Read the model definition and answer for the solid it produces. Units are mm, in the model's axes. Face numbers are marked on the shaded views. A direction names the side the tool comes from. Coordinates: 2 decimals unless noted, no trailing zeros. Order: outer loops, then holes, each group sorted by start corner. A loop starts at its lowest first (then second) coordinate and runs counter-clockwise, first axis right, second up. Notation, with made-up numbers: (21.25, 6.5) - (38.25, 6.5) arc R33 cw to (38.25, 42.5) - close; hole circle Ø4 at (79, -28.75). An arc over 180 degrees is marked (long way). Use one line per item in the form item = value.
```python
from build123d import *

# Parameters (mm, degrees)
BOSS_EXTRUDE2_DEPTH = 20
SKETCH2_R           = 3
CUT_EXTRUDE1_DEPTH  = 20
SKETCH3_W           = 200
SKETCH3_H           = 120
CUT_EXTRUDE2_DEPTH  = 10
FILLET1_R           = 5
BOSS_EXTRUDE3_START = -10
SKETCH6_R           = 3
SKETCH6_R_2         = 2.5
BOSS_EXTRUDE3_DEPTH = 10
SKETCH7_R           = 4.7
CUT_EXTRUDE6_DEPTH  = 5
SKETCH4_W           = 18
SKETCH4_H           = 81
CUT_EXTRUDE7_DEPTH  = 5


with BuildPart() as part:
    # Sketch1 → Boss-Extrude2 (new body)
    with BuildSketch(Plane.XY):
        Polygon((0, 0), (240, 0), (240, 10), (220, 10), (220, 130), (20, 130), (20, 10), (0, 10), align=None)
    extrude(amount=BOSS_EXTRUDE2_DEPTH)

    # Sketch2 → Cut-Extrude1 (cut)
    with BuildSketch(Plane(origin=(0, 10, 0), x_dir=(1, 0, 0), z_dir=(0, 1, 0))):
        with Locations(Location((10, -10, 0), (0, 0, 180))):
            Circle(SKETCH2_R)
        with Locations(Location((230, -10, 0), (0, 0, 180))):
            Circle(SKETCH2_R)
    extrude(amount=-CUT_EXTRUDE1_DEPTH, mode=Mode.SUBTRACT)

    # Sketch3 → Cut-Extrude2 (cut)
    with BuildSketch(Plane(origin=(0, 0, 0), x_dir=(-1, 0, 0), z_dir=(0, 0, -1))):
        with Locations((-120, 70)):
            Rectangle(SKETCH3_W, SKETCH3_H)
    extrude(amount=-CUT_EXTRUDE2_DEPTH, mode=Mode.SUBTRACT)

    # Fillet1
    fillet1_edges = [part.edges().sort_by_distance(p)[0] for p in [
        (120, 10, 10),
    ]]
    fillet(fillet1_edges, radius=FILLET1_R)

    # Sketch6 → Boss-Extrude3 (add)
    # profile 1 of 2: a face of its own
    with BuildSketch(Plane.XZ.offset(BOSS_EXTRUDE3_START)):
        with Locations((10, 10)):
            Circle(SKETCH6_R)
        with Locations(Location((10, 10, 0), (0, 0, 270))):
            Circle(SKETCH6_R_2, mode=Mode.SUBTRACT)
    # profile 2 of 2: a face of its own
    with BuildSketch(Plane.XZ.offset(BOSS_EXTRUDE3_START)):
        with Locations((230, 10)):
            Circle(SKETCH6_R)
        with Locations(Location((230, 10, 0), (0, 0, 270))):
            Circle(SKETCH6_R_2, mode=Mode.SUBTRACT)
    extrude(amount=BOSS_EXTRUDE3_DEPTH)

    # Sketch7 → Cut-Extrude6 (cut)
    with BuildSketch(Plane(origin=(0, 10, 0), x_dir=(1, 0, 0), z_dir=(0, 1, 0))):
        with Locations(Location((230, -10, 0), (0, 0, 180))):
            Circle(SKETCH7_R)
        with Locations(Location((10, -10, 0), (0, 0, 180))):
            Circle(SKETCH7_R)
    extrude(amount=-CUT_EXTRUDE6_DEPTH, mode=Mode.SUBTRACT)

    # Sketch4 → Cut-Extrude7 (cut)
    with BuildSketch(Plane.XY.offset(20)):
        with Locations((57, 69.5)):
            Rectangle(SKETCH4_W, SKETCH4_H)
        with Locations((183, 69.5)):
            Rectangle(SKETCH4_W, SKETCH4_H)
    extrude(amount=-CUT_EXTRUDE7_DEPTH, mode=Mode.SUBTRACT)


solid = part.part
```
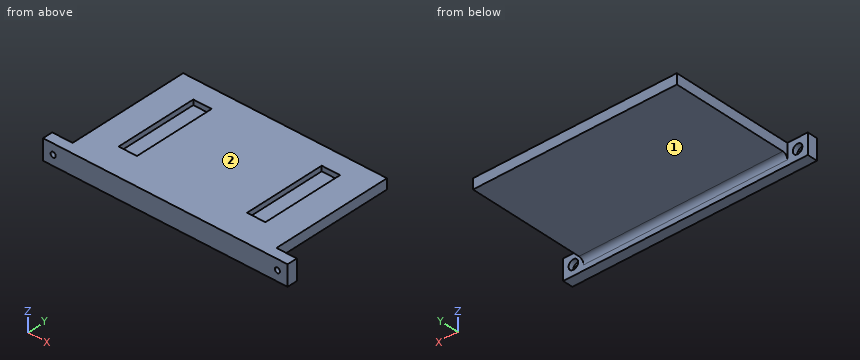
(1) Which of the six approach directions +Z, -Z, +X, -X, +Y, -Y give full straight-line access (tool end or side, diameter ignored) to the marked faces 1 and 2?
Answer list:
face_1 = -Z, +X, -X, +Y
face_2 = +Z, +X, -X, +Y, -Y
(2) Section D-D, the plane x = 94 is taken. Write down the section's boundary in (y, z).
Answer list:
outline = (0, 0) - (10, 0) - (10, 5) arc R5 cw to (15, 10) - (130, 10) - (130, 20) - (0, 20) - close
(3) Section B-B, the plane y = 74.5 is taken. Write down the section's boundary in (x, z).
Answer list:
outline = (20, 10) - (220, 10) - (220, 20) - (192, 20) - (192, 15) - (174, 15) - (174, 20) - (66, 20) - (66, 15) - (48, 15) - (48, 20) - (20, 20) - close
(4) Straight lines are drawn through the part: L1, parallel to X at y = 1.65, z = 10; L2, parallel to Z at x = 230, y = 6.9; L3, parallel to Z at x = 10, y = 3.75. For each, find the intervals that lie inside material, in ascending order.
Answer list:
L1 = 0 to 7.5, 12.5 to 227.5, 232.5 to 240
L2 = 0 to 5.3, 14.7 to 20
L3 = 0 to 7.5, 12.5 to 20
(5) Section A-A, the plane x = 10 is taken. Write down the section's boundary in (y, z).
Answer list:
outline = (0, 0) - (10, 0) - (10, 5.3) - (5, 5.3) - (5, 7.5) - (0, 7.5) - close; (0, 12.5) - (5, 12.5) - (5, 14.7) - (10, 14.7) - (10, 20) - (0, 20) - close
(6) Given pin 1 Ø1.5 at (y, z) = (87, 17) entering from +X; pin 2 Ø3 at (x, y) = (41, 75.5) entering from -Z; pin 3 Ø4 at (x, z) = (149.5, 3) entering from -Y; pin 4 Ø12 at (y, z) = (57.5, 10.5) entering from -X, each flat-ended and moving along its own axis, determine where each tip first touches the part or whether it passes through.
Answer list:
pin_1 = 220
pin_2 = 10
pin_3 = 0
pin_4 = 20
(7) Section C-C, the plane x = 179.5 is taken. Write down the section's boundary in (y, z).
Answer list:
outline = (0, 0) - (10, 0) - (10, 5) arc R5 cw to (15, 10) - (130, 10) - (130, 20) - (110, 20) - (110, 15) - (29, 15) - (29, 20) - (0, 20) - close
